from build123d import *

# Parameters (mm, degrees)
BOSS_EXTRUDE1_DEPTH = 25.4
SKETCH2_W           = 25.4
SKETCH2_H           = 1.524
BOSS_EXTRUDE2_DEPTH = 25.4
SKETCH5_R           = 1.5
CUT_EXTRUDE1_DEPTH  = 2.54


with BuildPart() as part:
    # Sketch1 → Boss-Extrude1 (new body)
    with BuildSketch(Plane(origin=(0, 0, 0), x_dir=(-1, 0, 0), z_dir=(0, 0, -1))):
        with BuildLine():
            Line((7.9375, 2.8575), (9.4615, 2.8575))
            Line((9.4615, 2.8575), (9.4615, 7.9375))
            ThreePointArc((9.4615, 7.9375), (1.5875, 15.8115), (-6.2865, 7.9375))
            Line((-6.2865, 7.9375), (-6.2865, 2.8575))
            Line((-6.2865, 2.8575), (-4.7625, 2.8575))
            Line((-4.7625, 2.8575), (-4.7625, 7.9375))
            ThreePointArc((-4.7625, 7.9375), (1.5875, 14.2875), (7.9375, 7.9375))
            Line((7.9375, 7.9375), (7.9375, 2.8575))
        make_face()
    extrude(amount=-BOSS_EXTRUDE1_DEPTH)

    # Sketch2 → Boss-Extrude2 (add)
    with BuildSketch(Plane.ZY.offset(9.4615)):
        with Locations((12.7, 3.6195)):
            Rectangle(SKETCH2_W, SKETCH2_H)
    extrude(amount=BOSS_EXTRUDE2_DEPTH)

    # Sketch5 → Cut-Extrude1 (cut)
    with BuildSketch(Plane(origin=(0, 4.3815, 0), x_dir=(1, 0, 0), z_dir=(0, 1, 0))):
        with Locations((-22.1615, -12.7)):
            Circle(SKETCH5_R)
    extrude(amount=-CUT_EXTRUDE1_DEPTH, mode=Mode.SUBTRACT)


solid = part.part
Check sheet for the modelled part. Datum: model origin and axes. Units: mm. A direction names the side the tool comes from. Round coordinates to 2 decimals unless told otherwise and drop trailing zeros. Order: outer loops, then holes, each group sorted by start corner. A loop starts at its lowest first (then second) coordinate and runs counter-clockwise, first axis right, second up.
(1) Go/stop test with flat-tipped pins: P1, Ø1.8, axis at y = 6, z = 16.5, coming from the -X side; P2, Ø1, axis at x = -17.5, z = 18.5, coming from the +Y side; P3, Ø2, axis at x = -4, z = 17.5, coming from the +Y side. Record where each tip stops, or that it passes through.
(2) Cross-section at B-B, the plane y = 13.5. Enter the section's corners in (x, z), and give its area (3 significant figures).
(3) Access from +Z, -Z, +X, -X, +Y, -Y to the whole of each face (thin tool, end or side, straight path). Record for faces 1 (the flat face through (-7.938, 5, 13)), 2 (the flat face through (6, 2.858, 13)), 3 (the flat face through (-25, 4.382, 13)).
(4) Draft check along X on faces 4 (the flat face through (6.286, 5, 13)), 5 (the flat face through (-21, 2.858, 15)), 6 (the flat face through (4.762, 5, 13)). Enter one of: pulls with the +X half, pulls with the -X half, needs draft (parallel to the pull), parting line crosses it, or undercut.
(5) Scan lines: probe 1 along X at (y, z) = (3.4, 12.7); probe 2 along X at (y, z) = (4.25, 5); probe 3 along Y at (x, z) = (-31.5, 7). Record each from-to range of solid material in increasing order.
(6) Cross-section at D-D, the plane y = 10.5. Enter the section's corners in (x, z).
(7) Cross-section at A-A, the plane z = 12.7. Enter the section's corners in (x, y), and give its area (3 significant figures).
(8) Cross-section at C-C, the plane z = 19. Enter the section's corners in (x, y).
Check sheet entries:
1. P1: stops at x = -9.46
1. P2: stops at y = 4.38
1. P3: stops at y = 15.68
2. outline: (-7.16, 0) - (-4.65, 0) - (-4.65, 25.4) - (-7.16, 25.4) - close; (1.48, 0) - (3.99, 0) - (3.99, 25.4) - (1.48, 25.4) - close
2. area: 128 mm2
3. face 1: +Z, -Z, -Y
3. face 2: +Z, -Z, +X, -X, -Y
3. face 3: +Z, -Z, -X, +Y
4. face 4: pulls with the +X half
4. face 5: needs draft
4. face 6: undercut
5. probe 1: x = -34.86 to -23.66, -20.66 to -7.94, 4.76 to 6.29
5. probe 2: x = -34.86 to -7.94, 4.76 to 6.29
5. probe 3: y = 2.86 to 4.38
6. outline: (-9.03, 0) - (-7.4, 0) - (-7.4, 25.4) - (-9.03, 25.4) - close; (4.22, 0) - (5.86, 0) - (5.86, 25.4) - (4.22, 25.4) - close
7. outline: (-34.86, 2.86) - (-23.66, 2.86) - (-23.66, 4.38) - (-34.86, 4.38) - close; (-20.66, 2.86) - (-7.94, 2.86) - (-7.94, 7.94) arc R6.35 cw to (4.76, 7.94) - (4.76, 2.86) - (6.29, 2.86) - (6.29, 7.94) arc R7.87 ccw to (-9.46, 7.94) - (-9.46, 4.38) - (-20.66, 4.38) - close
7. area: 83.7 mm2
8. outline: (-34.86, 2.86) - (-7.94, 2.86) - (-7.94, 7.94) arc R6.35 cw to (4.76, 7.94) - (4.76, 2.86) - (6.29, 2.86) - (6.29, 7.94) arc R7.87 ccw to (-9.46, 7.94) - (-9.46, 4.38) - (-34.86, 4.38) - close
